from build123d import *

# Parameters (mm, degrees)
SKETCH1_R           = 32.5
BOSS_EXTRUDE1_DEPTH = 10
SKETCH2_R           = 3
BOSS_EXTRUDE2_DEPTH = 70


with BuildPart() as part:
    # Sketch1 → Boss-Extrude1 (new body)
    with BuildSketch(Plane(origin=(0, 0, 0), x_dir=(1, 0, 0), z_dir=(0, 1, 0))):
        with BuildLine():
            ThreePointArc((-31.622776602, -7.5), (-25.495097568, 20.155644371), (0, 32.5))
            Line((0, 32.5), (-165, 32.5))
            Line((-165, 32.5), (-165, -7.5))
            Line((-165, -7.5), (-31.622776602, -7.5))
        make_face()
        Circle(SKETCH1_R)
    extrude(amount=BOSS_EXTRUDE1_DEPTH)

    # Sketch2 → Boss-Extrude2 (add)
    with BuildSketch(Plane(origin=(0, 10, 0), x_dir=(1, 0, 0), z_dir=(0, 1, 0))):
        with Locations(Location((0, 0, 0), (0, 0, 270))):
            Circle(SKETCH2_R)
    extrude(amount=BOSS_EXTRUDE2_DEPTH)


solid = part.part
Read the model definition and answer for the solid it produces. Units are mm, in the model's axes. A direction names the side the tool comes from. Give positions to 0.01 mm unless a question says otherwise; leave off trailing zeros. Write each loop counter-clockwise with the first axis right and the second up, starting at its lowest first coordinate (ties: lowest second). Pieces come first, ordered by that corner, then holes. Notation, with made-up numbers: (17.25, 2) - (44.25, 2) arc R31 ccw to (44.25, 27) - close; hole circle Ø8 at (2.5, 55.25). An arc over 180 degrees is marked (long way). Answer in a Markdown table with one row per item. Add a question column.
Item 1: A tool of negligible diameter and unlimited length cuts with its end or side. For faces 1 (the face through (-165, 5, -13)), 2 (the face through (-99, 5, 7.5)), 3 (the face through (0.9, 44.51, 2.86)), from which of +Z, -Z, +X, -X, +Y, -Y can it reach the whole face along a straight path? Write none if from no direction.
Item 2: Section A-A, the plane z = 0 is taken. Write down the section's boundary in (x, y), and give its area (4 significant figures).
Item 3: Section C-C, the plane x = -119.5 is taken. Write down the section's boundary in (y, z).
Item 4: Section D-D, the plane z = 16.5 is taken. Write down the section's boundary in (x, y), and give its area (3 significant figures).
Item 5: Flat-ended cylindrical pins translate along their axes: P1, Ø8, axis at x = -98.5, y = 6, coming from the +Z side; P2, Ø19.5, axis at x = -55, z = 11.5, coming from the +Y side. Find the tip coordinate at first contact, or state that the pin passes through.
Item 6: Section B-B, the plane y = 35 is taken. Write down the section's boundary in (x, z).
Item 7: Find the intervals of material crossed by L1, parallel to Y at x = -141, z = -25.5; L2, parallel to Z at x = -124.5, y = 7; L3, parallel to Z at x = -1, y = 51, in increasing order.
Recorded:
| question | item | result |
|---|---|---|
| 1 | face 1 | +Z, -Z, -X, +Y, -Y |
| 1 | face 2 | +Z, -X, +Y, -Y |
| 1 | face 3 | +Y |
| 2 | outline | (-165, 0) - (32.5, 0) - (32.5, 10) - (3, 10) - (3, 80) - (-3, 80) - (-3, 10) - (-165, 10) - close |
| 2 | area | 2,395 mm2 |
| 3 | outline | (0, -32.5) - (10, -32.5) - (10, 7.5) - (0, 7.5) - close |
| 4 | outline | (-28, 0) - (28, 0) - (28, 10) - (-28, 10) - close |
| 4 | area | 560 mm2 |
| 5 | P1 | stops at z = 7.5 |
| 5 | P2 | stops at y = 10 |
| 6 | outline | circle Ø6 at (0, 0) |
| 7 | L1 | y = 0 to 10 |
| 7 | L2 | z = -32.5 to 7.5 |
| 7 | L3 | z = -2.83 to 2.83 |
